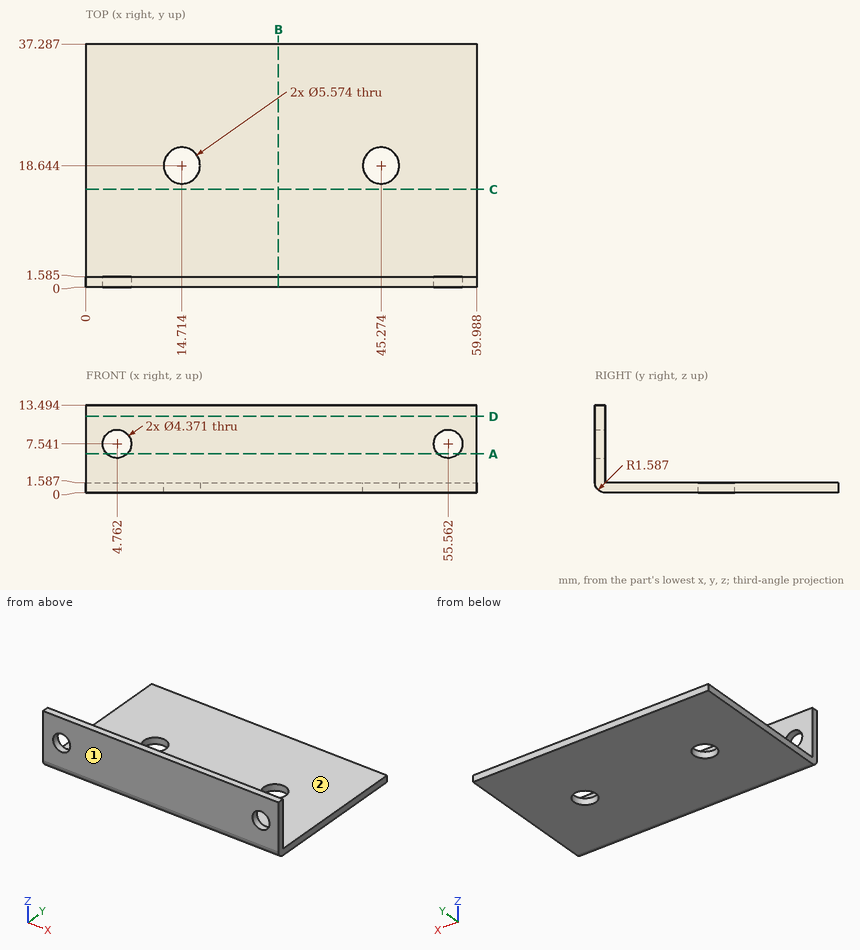
The drawing under review shows one solid part. Ordinate dimensions are in mm from its lowest x, y, z. A direction names the side the tool comes from. Coordinates: 2 decimals unless noted, no trailing zeros. Order: outer loops, then holes, each group sorted by start corner. A loop starts at its lowest first (then second) coordinate and runs counter-clockwise, first axis right, second up. Notation, with made-up numbers: (20, 15.5) -> (38, 15.5) arc R21 cw to (38, 51.5) -> close; hole circle Ø4 at (-33.5, 55). An arc over 180 degrees is marked (long way). Use CSV: the item, a comma, the result in double quotes. Start each with the question number.
Item 1: Insertion check: pin 1 (2 mm diameter, centred on x = 30, y = 9.5, fed in from +Z); pin 2 (5.5 mm diameter, centred on x = 55.56, z = 7.54, fed in from +Y) (1 decimal); pin 3 (5 mm diameter, centred on x = 45.27, y = 18.64, fed in from +Z). Each pin has a flat end and moves straight along its axis. Give the tip position at first contact, or say it passes through.
Item 2: For the marked faces 1 and 2, list the 3-axis set-ups (+Z, -Z, +X, -X, +Y, -Y) from which the entire face can be reached by the end or side of a thin tool; tool diameter is ignored.
Item 3: We need section C-C, the plane y = 15. Give the boundary of the cut face in (x, z).
Item 4: We need section D-D, the plane z = 11.75. Give the boundary of the cut face in (x, y) (1 decimal).
Item 5: Wall thickness on probe 1 along Z at (x, y) = (5.5, 16.5); probe 2 along Y at (x, z) = (55, 11.25) (1 decimal): over which ranges is each line inside the solid? List them lowest first.
Item 6: We need section A-A, the plane z = 6. Give the boundary of the cut face in (x, y) (1 decimal).
Item 7: We need section B-B, the plane x = 29.5. Give the boundary of the cut face in (y, z) (1 decimal).
Derived:
1,pin 1,"stops at z = 1.59"
1,pin 2,"stops at y = 1.6"
1,pin 3,"passes through"
2,face 1,"+Z, -Z, +X, -X, -Y"
2,face 2,"+Z, +X, -X, +Y"
3,outline,"(0, 0) -> (59.99, 0) -> (59.99, 1.59) -> (0, 1.59) -> close"
4,outline,"(0, 0) -> (60, 0) -> (60, 1.6) -> (0, 1.6) -> close"
5,probe 1,"z = 0 to 1.59"
5,probe 2,"y = 0 to 1.6"
6,outline,"(0, 0) -> (3.2, 0) -> (3.2, 1.6) -> (0, 1.6) -> close; (6.3, 0) -> (54, 0) -> (54, 1.6) -> (6.3, 1.6) -> close; (57.1, 0) -> (60, 0) -> (60, 1.6) -> (57.1, 1.6) -> close"
7,outline,"(0, 1.6) arc R1.6 ccw to (1.6, 0) -> (37.3, 0) -> (37.3, 1.6) -> (1.6, 1.6) -> (1.6, 13.5) -> (0, 13.5) -> close"
